from build123d import *

# Parameters (mm, degrees)
SKETCH1_R                = 2.1
BOSS_EXTRUDE1_DEPTH      = 3
BOSS_EXTRUDE1_DEPTH_BACK = 3
SKETCH2_R                = 4.55
CUT_EXTRUDE1_DEPTH       = 2.6
CHAMFER1_SIZE            = 1
CUT_EXTRUDE2_DEPTH       = 7
CHAMFER2_SIZE            = 0.5


with BuildPart() as part:
    # Sketch1 → Boss-Extrude1 (new body, two sides)
    with BuildSketch(Plane.XY) as boss_extrude1_sk:
        with BuildLine():
            Line((-39.501683147, 30.554976886), (14.53901549, 30.554976886))
            ThreePointArc((14.53901549, 30.554976886), (23.141239174, 24.201058459), (19.597278951, 14.110920817))
            ThreePointArc((19.597278951, 14.110920817), (12.655063172, 7.14488544), (8.796867444, -1.901347727))
            ThreePointArc((8.796867444, -1.901347727), (1.705655337, -8.836896507), (-7.457341048, -5.038657013))
            ThreePointArc((-7.457341048, -5.038657013), (-21.441099585, 7.679919061), (-39.703613005, 12.557242486))
            ThreePointArc((-39.703613005, 12.557242486), (-48.501116729, 21.65594817), (-39.501683147, 30.554976886))
        make_face()
        Circle(SKETCH1_R, mode=Mode.SUBTRACT)
        with Locations((-39.501683147, 21.554976886)):
            Circle(SKETCH1_R, mode=Mode.SUBTRACT)
        with Locations((14.53901549, 21.554976886)):
            Circle(SKETCH1_R, mode=Mode.SUBTRACT)
    extrude(amount=BOSS_EXTRUDE1_DEPTH)
    extrude(boss_extrude1_sk.sketch, amount=-BOSS_EXTRUDE1_DEPTH_BACK)

    # Sketch2 → Cut-Extrude1 (cut)
    with BuildSketch(Plane.XY.offset(3)):
        with Locations((-39.501683147, 21.554976886)):
            Circle(SKETCH2_R)
        with Locations((14.53901549, 21.554976886)):
            Circle(SKETCH2_R)
        Circle(SKETCH2_R)
    cut_extrude1 = extrude(amount=-CUT_EXTRUDE1_DEPTH, mode=Mode.SUBTRACT)

    # Mirror1: Cut-Extrude1 across plane
    add(cut_extrude1.mirror(Plane.XY), mode=Mode.SUBTRACT)

    # Chamfer1
    chamfer1_edges = [part.edges().sort_by_distance(p)[0] for p in [
        (1.705655337, -8.836896507, -3),
        (12.655063172, 7.14488544, -3),
        (23.141239174, 24.201058459, -3),
        (-12.481333828, 30.554976886, -3),
        (-48.501116729, 21.65594817, 3),
        (-21.441099585, 7.679919061, 3),
        (1.705655337, -8.836896507, 3),
        (12.655063172, 7.14488544, 3),
        (23.141239174, 24.201058459, 3),
        (-12.481333828, 30.554976886, 3),
        (-48.501116729, 21.65594817, -3),
        (-21.441099585, 7.679919061, -3),
    ]]
    chamfer(chamfer1_edges, length=CHAMFER1_SIZE)

    # Sketch3 → Cut-Extrude2 (cut, through all)
    with BuildSketch(Plane.XY.offset(3)):
        with BuildLine():
            Line((-24.180281108, 26.554976886), (-22.764342389, 26.554976886))
            ThreePointArc((-22.764342389, 26.554976886), (-21.583396496, 26.169091752), (-20.858160069, 25.160343686))
            Line((-20.858160069, 25.160343686), (-17.281431039, 13.89791957))
            ThreePointArc((-17.281431039, 13.89791957), (-17.903964164, 11.758849819), (-20.119238586, 11.522785996))
            ThreePointArc((-20.119238586, 11.522785996), (-23.13863628, 12.96831982), (-26.259194014, 14.180115968))
            ThreePointArc((-26.259194014, 14.180115968), (-30.454415742, 21.246945404), (-24.180281108, 26.554976886))
        make_face()
        with BuildLine():
            Line((-8.643875433, 24.622717198), (2.795841433, 20.183210519))
            ThreePointArc((2.795841433, 20.183210519), (4.612056387, 20.372573761), (5.51742454, 21.958387022))
            ThreePointArc((5.51742454, 21.958387022), (5.741336481, 23.592791168), (6.25883004, 25.159192739))
            ThreePointArc((6.25883004, 25.159192739), (6.178513352, 26.104179516), (5.344107869, 26.554976886))
            Line((5.344107869, 26.554976886), (-8.282085612, 26.554976886))
            ThreePointArc((-8.282085612, 26.554976886), (-9.265004655, 25.73901535), (-8.643875433, 24.622717198))
        make_face()
        with BuildLine():
            Line((-14.767813151, 19.218195089), (-10.2137058, 4.878196721))
            ThreePointArc((-10.2137058, 4.878196721), (-9.068134637, 3.935197355), (-7.738892439, 4.594512359))
            ThreePointArc((-7.738892439, 4.594512359), (-2.798782744, 8.553760293), (3.526217449, 8.280446274))
            ThreePointArc((3.526217449, 8.280446274), (8.030102489, 10.136580166), (6.10124738, 14.609803998))
            Line((6.10124738, 14.609803998), (-12.138051189, 21.688081264))
            ThreePointArc((-12.138051189, 21.688081264), (-14.230835601, 21.281395314), (-14.767813151, 19.218195089))
        make_face()
    extrude(amount=-CUT_EXTRUDE2_DEPTH, mode=Mode.SUBTRACT)

    # Chamfer2
    chamfer2_edges = [part.edges().sort_by_distance(p)[0] for p in [
        (-23.13863628, 12.96831982, -3),
        (-30.454415742, 21.246945404, -3),
        (-23.472311748, 26.554976886, -3),
        (-21.583396496, 26.169091752, -3),
        (-19.069795554, 19.529131628, -3),
        (-17.903964164, 11.758849819, -3),
        (-23.13863628, 12.96831982, 3),
        (-17.903964164, 11.758849819, 3),
        (-19.069795554, 19.529131628, 3),
        (-21.583396496, 26.169091752, 3),
        (-23.472311748, 26.554976886, 3),
        (-30.454415742, 21.246945404, 3),
        (4.612056387, 20.372573761, -3),
        (-2.924017, 22.402963859, -3),
        (-9.265004655, 25.73901535, -3),
        (-1.468988872, 26.554976886, -3),
        (6.178513352, 26.104179516, -3),
        (5.741336481, 23.592791168, -3),
        (4.612056387, 20.372573761, 3),
        (5.741336481, 23.592791168, 3),
        (6.178513352, 26.104179516, 3),
        (-1.468988872, 26.554976886, 3),
        (-9.265004655, 25.73901535, 3),
        (-2.924017, 22.402963859, 3),
        (-9.068134637, 3.935197355, -3),
        (-12.490759475, 12.048195905, -3),
        (-14.230835601, 21.281395314, -3),
        (-3.018401905, 18.148942631, -3),
        (8.030102489, 10.136580166, -3),
        (-2.798782744, 8.553760293, -3),
        (-9.068134637, 3.935197355, 3),
        (-2.798782744, 8.553760293, 3),
        (8.030102489, 10.136580166, 3),
        (-3.018401905, 18.148942631, 3),
        (-14.230835601, 21.281395314, 3),
        (-12.490759475, 12.048195905, 3),
    ]]
    chamfer(chamfer2_edges, length=CHAMFER2_SIZE)


solid = part.part
Work out the finished part from the listing and answer in its coordinate system (mm). A direction names the side the tool comes from. Give positions to 0.01 mm unless a question says otherwise; leave off trailing zeros. Use a Markdown table: item, result. Add a question column.
1) Which of the six approach directions +Z, -Z, +X, -X, +Y, -Y give full straight-line access (tool end or side, diameter ignored) to faces 4 (the flat face through (-2.89, 18.1, 0.03)), 5 (the cylindrical face through (18.74, 19.81, -1.72)), 6 (the cylindrical face through (-0.99, -4.44, 1.72))?
2) Consider line 1 along Y through (x, z) = (0, 2); line 2 along Y through (x, z) = (-0.5, -0.25); line 3 along Y through (x, z) = (-5, -1). Determine where each line is inside the solid, lowest interval first.
3) The part is cut by section A-A, the plane x = -1. Count the separate pieces of the cut face and the enclosed holes in it, plus the area to 3 significant figures.
4) Each of these flat-tipped pins is pushed along its axis until it touches: P1, Ø12, axis at x = 0, y = 0, coming from the -Z side; P2, Ø2.5, axis at x = -1, y = 0.5, coming from the -Z side; P3, Ø2, axis at y = 1.5, z = 1, coming from the -X side; P4, Ø1.5, axis at y = -1.5, z = -2, coming from the -X side. Where does it stop, or does it pass through?
5) For a pull along X with two mould halves and no side action, classify faces 1 (the cylindrical face through (12.733, 7.26, 0.028)), 2 (the flat face through (-10, 22, -3)), 3 (the flat face through (-12.76, 12.07, -2.75)) as +X half, -X half, draft (parallel to the pull), parting line (faces both ways), or undercut.
Reported:
| question | item | result |
|---|---|---|
| 1 | face 4 | +Z, -Z |
| 1 | face 5 | -Z |
| 1 | face 6 | +Z |
| 2 | line 1 | y = -9 to -4.55, 4.55 to 9, 16.98 to 21.27, 26.55 to 30.55 |
| 2 | line 2 | y = -8.99 to -2.04, 2.04 to 8.99, 17.17 to 21.46, 26.55 to 30.55 |
| 2 | line 3 | y = -7.48 to 7.48, 18.92 to 23.21, 26.55 to 30.55 |
| 3 | separate pieces | 4 |
| 3 | enclosed holes | 0 |
| 3 | area | 105 mm^2 |
| 4 | P1 | stops at z = -3 |
| 4 | P2 | stops at z = -0.4 |
| 4 | P3 | stops at x = -14.07 |
| 4 | P4 | stops at x = -10.8 |
| 5 | face 1 | +X half |
| 5 | face 2 | draft |
| 5 | face 3 | undercut |
